Could you check a few things on this drawing? It's one solid part, dimensions in mm from its lowest x, y, z. A direction names the side the tool comes from. Give positions to 0.01 mm unless a question says otherwise; leave off trailing zeros. Loops run counter-clockwise (first coordinate to the right, second up) from the corner with the lowest first, then second, coordinate; pieces in that order, holes last. Notation, with made-up numbers: M 12,-18.5 L 18,-18.5 A18 cw 18,3.5 Z; hole C 66,54 d10. An arc over 180 degrees is marked long. Return JSON: item names as keys, results as strings. Group by question number.
1. For pin 1 (0.9 mm diameter, centred on x = 5, y = 3, fed in from +Z); pin 2 (1.5 mm diameter, centred on x = 13, y = 24.5, fed in from +Z); pin 3 (1.9 mm diameter, centred on x = 6, y = 36, fed in from -Z), each with a flat end and sliding along its axis, tell me the tip position at first contact or that it passes through.
2. Please list where these lines run through material, in increasing order: line 1 (Y direction, x = 6, z = 1.9); line 2 (X direction, y = 36, z = 1.35); line 3 (Y direction, x = 1.25, z = 1.5).
3. If we section it at A-A (z = 2.25): Write out the boundary of the cut face in (x, y), plus the area to 3 significant figures.
4. If we section it at B-B (x = 6): Write out the boundary of the cut face in (y, z), plus the area to 3 significant figures.
5. If we section it at C-C (y = 36): Write out the boundary of the cut face in (x, z), plus the area to 3 significant figures.
6. For the marked faces 4 and 5, which set-ups out of +Z, -Z, +X, -X, +Y, -Y let a thin tool reach every point of the face, with its end or its side?
7. If we section it at D-D (z = 7.25): Write out the boundary of the cut face in (x, y).
8. If we mould it in two halves opening along Y, with no side actions, what happens to the marked faces 1, 2 and 3? For each: +Y half, -Y half, draft (parallel to the pull), parting line (faces both ways), or undercut.
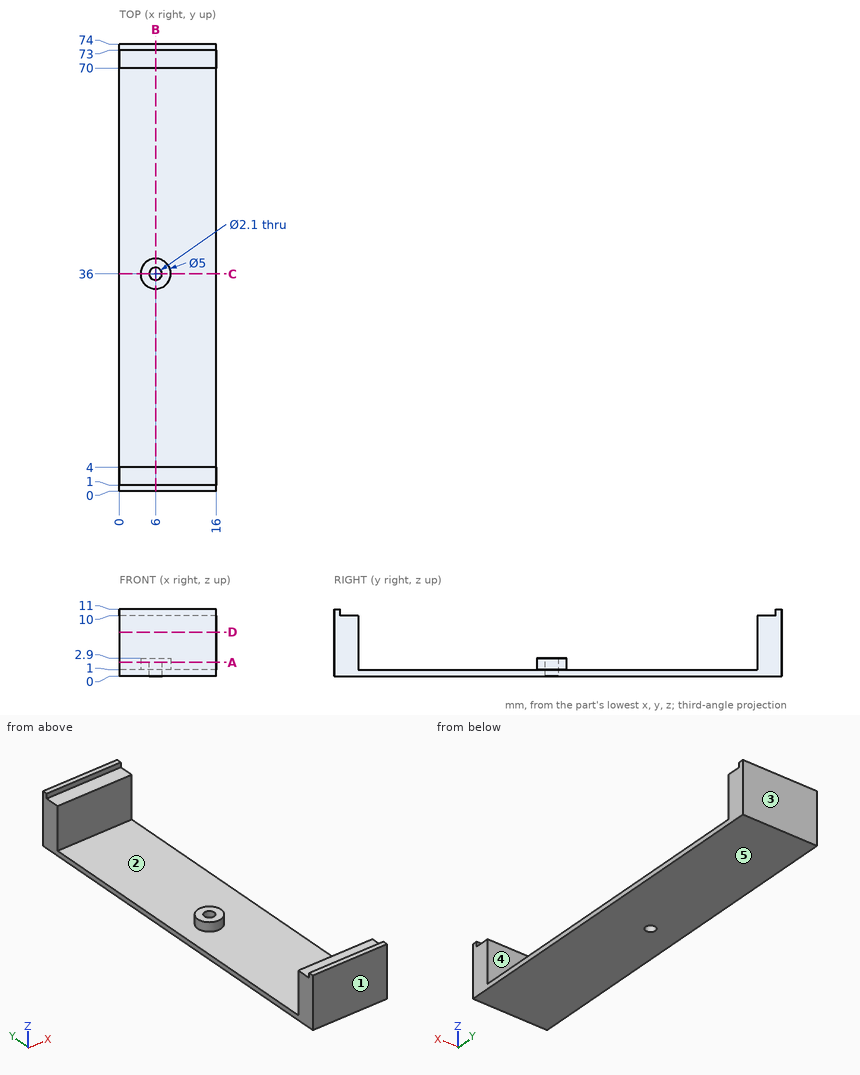
Answer:
{
 "1": {"pin 1": "stops at z = 10", "pin 2": "stops at z = 1", "pin 3": "passes through"},
 "2": {"line 1": "y = 0 to 4, 33.5 to 34.95, 37.05 to 38.5, 70 to 74", "line 2": "x = 3.5 to 4.95, 7.05 to 8.5", "line 3": "y = 0 to 4, 70 to 74"},
 "3": {"outline": "M 0,0 L 16,0 L 16,4 L 0,4 Z; M 0,70 L 16,70 L 16,74 L 0,74 Z; C 6,36 d5; hole C 6,36 d2.1", "area": "144 mm²"},
 "4": {"outline": "M 0,0 L 34.95,0 L 34.95,2.9 L 33.5,2.9 L 33.5,1 L 4,1 L 4,10 L 1,10 L 1,11 L 0,11 Z; M 37.05,0 L 74,0 L 74,11 L 73,11 L 73,10 L 70,10 L 70,1 L 38.5,1 L 38.5,2.9 L 37.05,2.9 Z", "area": "151 mm²"},
 "5": {"outline": "M 0,0 L 4.95,0 L 4.95,2.9 L 3.5,2.9 L 3.5,1 L 0,1 Z; M 7.05,0 L 16,0 L 16,1 L 8.5,1 L 8.5,2.9 L 7.05,2.9 Z", "area": "19.4 mm²"},
 "6": {"face 4": "+Z, +X, -X", "face 5": "-Z, +X, -X, +Y, -Y"},
 "7": {"outline": "M 0,0 L 16,0 L 16,4 L 0,4 Z; M 0,70 L 16,70 L 16,74 L 0,74 Z"},
 "8": {"face 1": "-Y half", "face 2": "undercut", "face 3": "+Y half"}
}
